Design review of the part built by this model. Coordinates are the model's own, in mm. Face numbers are marked on the shaded views. Give positions to 0.01 mm unless a question says otherwise; leave off trailing zeros. Write each loop counter-clockwise with the first axis right and the second up, starting at its lowest first coordinate (ties: lowest second). Pieces come first, ordered by that corner, then holes. Notation, with made-up numbers: (37, 52.5) -> (92, 52.5) arc R21 ccw to (92, 64.5) -> close; hole circle Ø6 at (-3.5, 32). An arc over 180 degrees is marked (long way). Return JSON: item names as keys, results as strings. Group by question number.
from build123d import *

# Parameters (mm, degrees)
F0_R      = 16.9164
F0_R_2    = 14.1605
F1_DEPTH  = 73.0504
F3_DEPTH  = 58.42
F5_DEPTH  = 25.4
F6_R      = 1.9304
F7_DEPTH  = 25.4
F8_R      = 1.9304
F9_DEPTH  = 35.814
F10_R     = 1.9304
F11_DEPTH = 25.4
F12_R     = 1.9304
F13_DEPTH = 44.196


with BuildPart() as f1:
    # F0 (on Top) → F1 (new body)
    with BuildSketch(Plane.XY):
        Circle(F0_R)
        Circle(F0_R_2, mode=Mode.SUBTRACT)
    extrude(amount=F1_DEPTH)

    # F2 (on Right) → F3 (cut)
    with BuildSketch(Plane.YZ):
        Polygon((-18.284496, 78.388058), (-18.916648, 7.546794), (19.261749, 78.388058), align=None)
    extrude(amount=F3_DEPTH, mode=Mode.SUBTRACT)

    # F4 (on Right) → F5 (cut)
    with BuildSketch(Plane.YZ):
        Polygon((-19.360213, 79.200871), (18.200016, 8.959677), (23.540258, 79.200871), align=None)
    extrude(amount=-F5_DEPTH, mode=Mode.SUBTRACT)

    # F6 (on Right) → F7 (cut)
    with BuildSketch(Plane.YZ):
        with Locations((0, 3.939143)):
            Circle(F6_R)
    extrude(amount=-F7_DEPTH, mode=Mode.SUBTRACT)

    # F8 (on Right) → F9 (cut)
    with BuildSketch(Plane.YZ):
        with Locations((0, 3.940872)):
            Circle(F8_R)
    extrude(amount=F9_DEPTH, mode=Mode.SUBTRACT)

    # F10 (on Front) → F11 (cut)
    with BuildSketch(Plane.XZ):
        with Locations((0, 4.125499)):
            Circle(F10_R)
    extrude(amount=-F11_DEPTH, mode=Mode.SUBTRACT)

    # F12 (on Front) → F13 (cut)
    with BuildSketch(Plane.XZ):
        with Locations((0, 4.12201)):
            Circle(F12_R)
    extrude(amount=F13_DEPTH, mode=Mode.SUBTRACT)


solid = f1.part
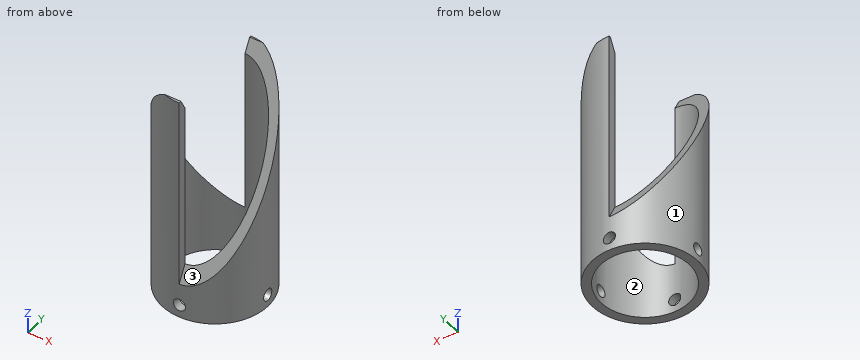
Q1. Take a section at D-D, the plane y = -5. Give the boundary of the cut face in (x, z).
Q2. Mouldability with a two-part tool opening along Y and no side actions: class the marked faces 1, 2 and 3 as +Y half, -Y half, draft (parallel to the pull), parting line (faces both ways), or undercut.
Q3. For L1, parallel to X at y = 0, z = 17; L2, parallel to Y at x = 8.5, z = 18.5; L3, parallel to X at y = 15, z = 5.5, list the stretches that pass through material, from the lowest coordinate up. Write a range as from..to.
Q4. Insertion check: pin 1 (8 mm diameter, centred on x = 13, z = 64.5, fed in from +Y); pin 2 (1 mm diameter, centred on x = -5, y = -13, fed in from +Z); pin 3 (2 mm diameter, centred on x = -3.5, z = 58, fed in from +Y). Each pin has a flat end and moves straight along its axis. Give the tip position at first contact, or say it passes through.
Q5. Take a section at C-C, the plane x = -4. Give the boundary of the cut face in (y, z), plus the area to 3 significant figures.
Q6. Take a section at A-A, the plane z = 44. Give the boundary of the cut face in (x, y), plus the area to 3 significant figures.
Q7. Take a section at B-B, the plane y = 0. Give the boundary of the cut face in (x, z).
Final values:
{
 "1": {"outline": "(-16.16, 0) -> (-13.25, 0) -> (-13.25, 52.35) -> (-16.16, 52.35) -> close; (13.25, 0) -> (16.16, 0) -> (16.16, 33.37) -> (13.25, 33.37) -> close"},
 "2": {"face 1": "parting line", "face 2": "undercut", "face 3": "-Y half"},
 "3": {"L1": "x = -16.92..-14.16, 14.16..16.92", "L2": "y = -13.01..-11.33, 11.33..14.63", "L3": "x = -7.82..-1.36, 1.36..7.82"},
 "4": {"pin 1": "stops at y = 14.32", "pin 2": "stops at z = 68.24", "pin 3": "stops at y = -13.43"},
 "5": {"outline": "(-16.44, 0) -> (-13.58, 0) -> (-13.58, 68.4) -> (-16.07, 73.05) -> (-16.44, 73.05) -> close; (13.58, 0) -> (16.44, 0) -> (16.44, 12.26) -> (13.58, 17.59) -> close", "area": "245 mm²"},
 "6": {"outline": "(-16.91, -0.54) arc R16.92 ccw to (0, -16.92) -> (0, -14.16) arc R14.16 cw to (-14.15, -0.54) -> close; (0, 14.16) arc R14.16 cw to (14.14, 0.73) -> (16.9, 0.73) arc R16.92 ccw to (0, 16.92) -> close", "area": "131 mm²"},
 "7": {"outline": "(-16.92, 0) -> (-14.16, 0) -> (-14.16, 2.01) -> (-16.92, 2.01) -> close; (-16.92, 5.87) -> (-14.16, 5.87) -> (-14.16, 43) -> (-16.92, 43) -> close; (14.16, 0) -> (16.92, 0) -> (16.92, 2.01) -> (14.16, 2.01) -> close; (14.16, 5.87) -> (16.92, 5.87) -> (16.92, 42.65) -> (14.16, 42.65) -> close"}
}
